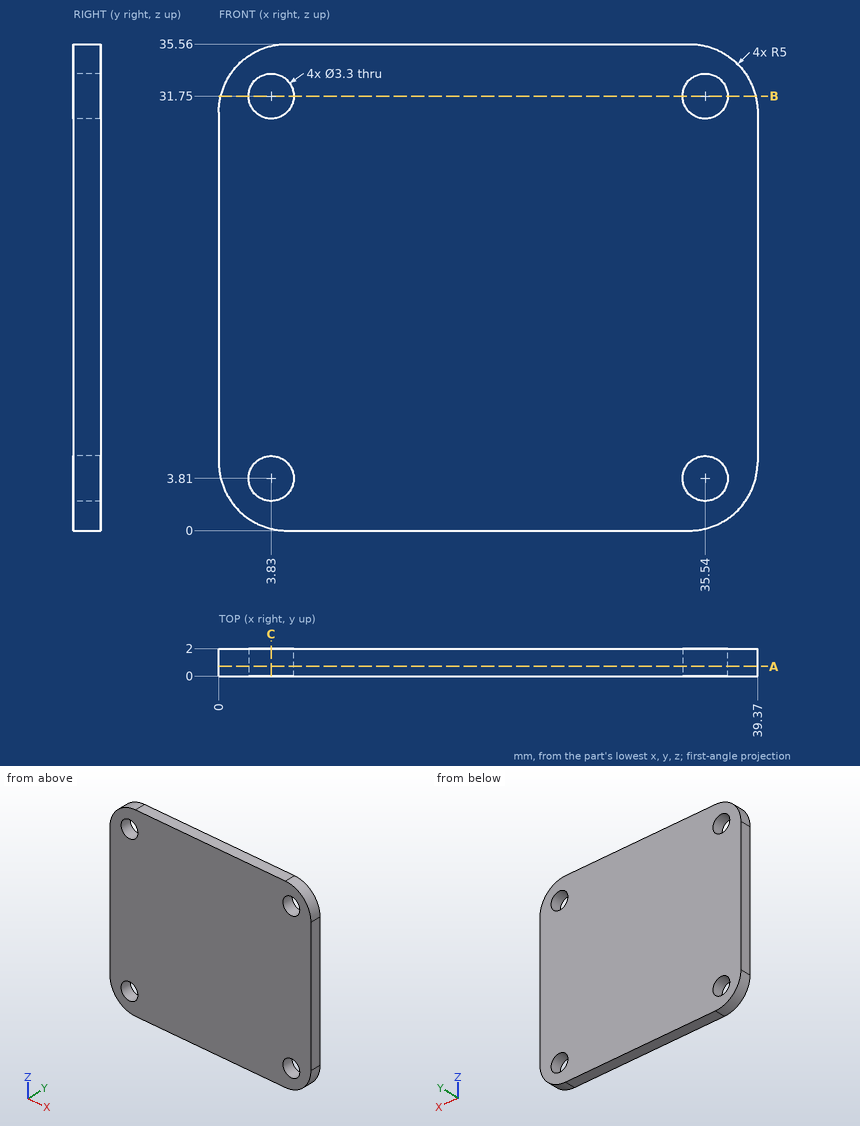
The figure shows three views and two pictorial views of one solid part (mm, origin at its lowest corner). Answer the questions. Give positions to 0.01 mm unless a question says otherwise; leave off trailing zeros. Write each loop counter-clockwise with the first axis right and the second up, starting at its lowest first coordinate (ties: lowest second). Pieces come first, ordered by that corner, then holes. Notation, with made-up numbers: (19.25, -32) - (25.25, -32) arc R19 ccw to (25.25, -13) - close; hole circle Ø2 at (-26.5, -38.75). An arc over 180 degrees is marked (long way). Use one line per item in the form item = value.
1. This flat-tipped pin is pushed along its axis until it touches: pin 1 Ø2 at (x, z) = (19, 27.5) entering from -Y. Where does it stop, or does it pass through?
Filled in:
pin_1 = 0
2. Consider L1, parallel to Z at x = 35.54, y = 1.35; L2, parallel to Z at x = 36, y = 1.5; L3, parallel to X at y = 1.3, z = 31.75. Determine where each line is inside the solid, lowest interval first.
Filled in:
L1 = 0.14 to 2.16, 5.46 to 30.1, 33.4 to 35.42
L2 = 0.27 to 2.23, 5.39 to 30.17, 33.33 to 35.29
L3 = 0.14 to 2.18, 5.48 to 33.89, 37.19 to 39.23
3. A cutting plane is placed at B-B (z = 31.75). Write down the section's boundary in (x, y), and give its area (3 significant figures).
Filled in:
outline = (0.14, 0) - (2.18, 0) - (2.18, 2) - (0.14, 2) - close; (5.48, 0) - (33.89, 0) - (33.89, 2) - (5.48, 2) - close; (37.19, 0) - (39.23, 0) - (39.23, 2) - (37.19, 2) - close
area = 65.0 mm^2
4. A cutting plane is placed at C-C (x = 3.83). Write down the section's boundary in (y, z), and give its area (3 significant figures).
Filled in:
outline = (0, 0.14) - (2, 0.14) - (2, 2.16) - (0, 2.16) - close; (0, 5.46) - (2, 5.46) - (2, 30.1) - (0, 30.1) - close; (0, 33.4) - (2, 33.4) - (2, 35.42) - (0, 35.42) - close
area = 57.4 mm^2
5. A cutting plane is placed at A-A (y = 0.7). Write down the section's boundary in (x, z), and give its area (3 significant figures).
Filled in:
outline = (0, 5) arc R5 ccw to (5, 0) - (34.37, 0) arc R5 ccw to (39.37, 5) - (39.37, 30.56) arc R5 ccw to (34.37, 35.56) - (5, 35.56) arc R5 ccw to (0, 30.56) - close; hole circle Ø3.3 at (3.83, 3.81); hole circle Ø3.3 at (3.83, 31.75); hole circle Ø3.3 at (35.54, 3.81); hole circle Ø3.3 at (35.54, 31.75)
area = 1,340 mm^2
